Autodesk Inventor part; units mm, degrees
ref_plane "YZ Plane" through (0, 0, 0) normal (1, 0, 0) x (0, 1, 0)
ref_plane "XZ Plane" through (0, 0, 0) normal (0, 1, 0) x (-1, 0, 0)
ref_plane "XY Plane" through (0, 0, 0) normal (0, 0, 1) x (1, 0, 0)
sketch "Sketch1" plane through (0, 0, 0) normal (0, 1, 0) x (-1, 0, 0)
  line L0 (-21.5, -3) -> (21.5, -3)
  line L1 (21.5, -3) -> (21.5, 3)
  line L2 (21.5, 3) -> (-21.5, 3)
  line L3 (-21.5, 3) -> (-21.5, -3)
  line L4 (-21.5, -3) -> (21.5, 3) construction
  line L5 (21.5, -3) -> (-21.5, 3) construction
  circle A0 centre (21.5, 0) radius 3
  circle A1 centre (-21.5, 0) radius 3
  point P0 (0, 0)
  dimension "d0" = 43
  dimension "d1" = 6
extrude "Extrusion1" add sketch "Sketch1" along normal blind 2
sketch "Sketch2" plane through (0, 2, 0) normal (0, 1, 0) x (1, 0, 0)
  arc A0 (21.5, -3) -> (21.5, 3) centre (21.5, 0) ccw
  arc A1 (-21.5, 3) -> (-21.5, -3) centre (-21.5, 0) ccw
  circle A2 centre (-21.5, 0) radius 1.5
  circle A3 centre (21.5, 0) radius 1.5
  point P0 (0, 0)
  dimension "d5" = 3
  dimension "d6" = 3
extrude "Extrusion2" cut sketch "Sketch2" against normal blind 2
sketch "Sketch3" plane through (0, 0, 0) normal (0, -1, 0) x (1, 0, 0)
  circle A0 centre (-21.5, 0) radius 1.5
  circle A1 centre (21.5, 0) radius 1.5
  arc A2 (21.5, -3) -> (21.5, 3) centre (21.5, 0) ccw
  arc A3 (-21.5, 3) -> (-21.5, -3) centre (-21.5, 0) ccw
  circle A4 centre (-21.5, 0) radius 0.05
  circle A5 centre (21.5, 0) radius 0.05
  point P0 (0, 0)
  dimension "d9" = 0.1
  dimension "d10" = 0.1
extrude "Extrusion3" add sketch "Sketch3" against normal blind 2
sketch "Sketch4" plane through (0, 0, 0) normal (0, -1, 0) x (1, 0, 0)
  circle A0 centre (-21.5, 0) radius 0.05
  circle A1 centre (21.5, 0) radius 0.05
  arc A2 (21.5, -3) -> (21.5, 3) centre (21.5, 0) ccw
  arc A3 (-21.5, 3) -> (-21.5, -3) centre (-21.5, 0) ccw
  circle A4 centre (-21.5, 0) radius 1.5
  circle A5 centre (21.5, 0) radius 1.5
  point P0 (0, 0)
  dimension "d13" = 3
  dimension "d14" = 3
extrude "Extrusion4" cut sketch "Sketch4" against normal blind 2
properties part number "tahlo7"
For this review, take the finished solid that the model builds, in its own axes (mm). Coordinates: 2 decimals unless noted, no trailing zeros. Write each loop counter-clockwise with the first axis right and the second up, starting at its lowest first coordinate (ties: lowest second). Pieces come first, ordered by that corner, then holes. Notation, with made-up numbers: (-35, 1.5) -> (-13, 1.5) arc R36 ccw to (-13, 40.5) -> close; hole circle Ø6 at (0.25, 63). An arc over 180 degrees is marked (long way). Put each result on its own line as item: value.
Q1. Take a section at C-C, the plane z = -2.6. State the section outline as (x, y) points.
From the geometry:
outline: (-23, 0) -> (23, 0) -> (23, 2) -> (-23, 2) -> close
Q2. Wall thickness on L1, parallel to Z at x = -21.5, y = 1.4; L2, parallel to X at y = 1.2, z = 0.4; L3, parallel to X at y = 0.15, z = -0.8: over which ranges is each line inside the solid? List them lowest first.
From the geometry:
L1: z = -3 to -1.5, 1.5 to 3
L2: x = -24.47 to -22.95, -20.05 to 20.05, 22.95 to 24.47
L3: x = -24.39 to -22.77, -20.23 to 20.23, 22.77 to 24.39
Q3. Take a section at B-B, the plane y = 0.95. State the section outline as (x, z) points, then the cut area to 3 significant figures.
From the geometry:
outline: (-21.5, -3) -> (21.5, -3) arc R3 ccw to (21.5, 3) -> (-21.5, 3) arc R3 ccw to start; hole circle Ø3 at (-21.5, 0); hole circle Ø3 at (21.5, 0)
area: 272 mm2
Q4. Take a section at A-A, the plane z = -0.55. State the section outline as (x, y) points, then the cut area to 3 significant figures.
From the geometry:
outline: (-24.45, 0) -> (-22.9, 0) -> (-22.9, 2) -> (-24.45, 2) -> close; (-20.1, 0) -> (20.1, 0) -> (20.1, 2) -> (-20.1, 2) -> close; (22.9, 0) -> (24.45, 0) -> (24.45, 2) -> (22.9, 2) -> close
area: 86.6 mm2
Q5. The part is to be moulded in two halves that separate along Z. For faces 1 (the flat face through (0, 2, 0)), 2 (the cylindrical face through (-24.5, 1, 0.1)), 3 (the cylindrical face through (-23, 1, 0)), say which applies: +Z half, -Z half, draft (parallel to the pull), parting line (faces both ways), or undercut.
From the geometry:
face 1: draft
face 2: parting line
face 3: undercut
